Design review of the part built by this model. Coordinates are the model's own, in mm. Face numbers are marked on the shaded views. A direction names the side the tool comes from. Coordinates: 2 decimals unless noted, no trailing zeros. Order: outer loops, then holes, each group sorted by start corner. A loop starts at its lowest first (then second) coordinate and runs counter-clockwise, first axis right, second up. Notation, with made-up numbers: (-31, 35.5) -> (-15, 35.5) arc R28 cw to (-15, 58.5) -> close; hole circle Ø1 at (65.5, 11.5). An arc over 180 degrees is marked (long way). Write item = value, one per line.
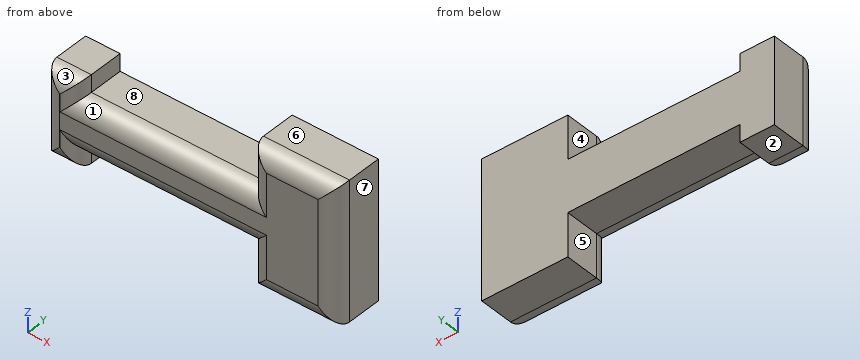
```python
from build123d import *

# Parameters (mm, degrees)
BOSS_EXTRUDE1_DEPTH = 3
FILLET2_R           = 1


with BuildPart() as part:
    # Sketch1 → Boss-Extrude1 (new body)
    with BuildSketch(Plane(origin=(0, 0, 0), x_dir=(1, 0, 0), z_dir=(0, 1, 0))):
        Polygon((-12.5, -1.5), (-12.5, -2.5), (-14.5, -2.5), (-14.5, 2.5), (-12.5, 2.5), (-12.5, 1.5), (-2.5, 1.5), (-2.5, 4), (2.5, 4), (2.5, -4), (-2.5, -4), (-2.5, -1.5), align=None)
    extrude(amount=BOSS_EXTRUDE1_DEPTH)

    # Fillet2
    fillet2_edges = [part.edges().sort_by_distance(p)[0] for p in [
        (0, 0, 4),
        (-2.5, 0, 2.75),
        (-7.5, 0, 1.5),
        (-12.5, 0, 2),
        (-13.5, 0, 2.5),
        (-14.5, 0, 0),
        (-13.5, 0, -2.5),
        (-12.5, 0, -2),
        (-7.5, 0, -1.5),
        (-2.5, 0, -2.75),
        (0, 0, -4),
        (2.5, 0, 0),
    ]]
    fillet(fillet2_edges, radius=FILLET2_R - 0.0001)  # a hair under: the kernel refuses the full size


solid = part.part
```
(1) We need section D-D (x = -12.25). Write out the cut boundary in (y, z).
Report:
outline = (0, -0.5) arc R1 ccw to (1, -1.5) -> (3, -1.5) -> (3, 1.5) -> (1, 1.5) arc R1 ccw to (0, 0.5) -> close
(2) We need section A-A (y = 1.55). Write out the cut boundary in (x, z).
Report:
outline = (-14.5, -2.5) -> (-12.5, -2.5) -> (-12.5, -1.5) -> (-2.5, -1.5) -> (-2.5, -4) -> (2.5, -4) -> (2.5, 4) -> (-2.5, 4) -> (-2.5, 1.5) -> (-12.5, 1.5) -> (-12.5, 2.5) -> (-14.5, 2.5) -> close
(3) For the marked faces 1, 2, 3, 4 and 5, list the 3-axis set-ups (+Z, -Z, +X, -X, +Y, -Y) from which the entire face can be reached by the end or side of a thin tool; tool diameter is ignored.
Report:
face_1 = +Z, -Y
face_2 = -Z, -X, +Y, -Y
face_3 = +Z, -X, -Y
face_4 = +Z, +Y, -Y
face_5 = -Z, +Y, -Y
(4) The part is to be moulded in two halves that separate along X. For the marked faces 6, 7 and 8, say which applies: released by +X, released by -X, zero draft, split by the parting line, or undercut.
Report:
face_6 = zero draft
face_7 = released by +X
face_8 = undercut
(5) Insertion check: pin 1 (1 mm diameter, centred on y = 1.5, z = 3.5, fed in from -X); pin 2 (4 mm diameter, centred on x = -10, z = -2.5, fed in from -Y); pin 3 (1.6 mm diameter, centred on x = -13.5, y = 2, fed in from +Z); pin 4 (1 mm diameter, centred on x = -13, y = 2.5, fed in from -Z). Each pin has a flat end and moves straight along its axis. Give the tip position at first contact, or say it passes through.
Report:
pin_1 = -2.5
pin_2 = 0
pin_3 = 2.5
pin_4 = -2.5
(6) We need section B-B (x = -0.5). Write out the cut boundary in (y, z).
Report:
outline = (0, -3) arc R1 ccw to (1, -4) -> (3, -4) -> (3, 4) -> (1, 4) arc R1 ccw to (0, 3) -> close
(7) For L1, parallel to X at y = 0.5, z = 1.75; L2, parallel to Z at x = -6.5, y = 2.3; L3, parallel to X at y = 2.25, z = 3.25, list the stretches that pass through material, from the lowest coordinate up.
Report:
L1 = -14.37 to -12.63, -2.37 to 2.37
L2 = -1.5 to 1.5
L3 = -2.5 to 2.5
